Can you work these out from the model? Positions are in its coordinate system, mm. A direction names the side the tool comes from. Give positions to 0.01 mm unless a question says otherwise; leave off trailing zeros. Order: outer loops, then holes, each group sorted by start corner. A loop starts at its lowest first (then second) coordinate and runs counter-clockwise, first axis right, second up. Notation, with made-up numbers: M -28.75,-10.75 L 3.25,-10.75 A26 cw 3.25,25.25 Z; hole C -5.5,2.5 d4. An arc over 180 degrees is marked long. Use a Markdown table: item, result. Add a question column.
from build123d import *

# Parameters (mm, degrees)
SALIENTE_EXTRUIR1_DEPTH = 3
REDONDEO1_R             = 35
CROQUIS2_W              = 3
CROQUIS2_H              = 33
CORTAR_EXTRUIR1_DEPTH   = 4
CROQUIS3_W              = 11.5
CROQUIS3_H              = 13
CORTAR_EXTRUIR2_DEPTH   = 4
CROQUIS4_W              = 12
CROQUIS4_H              = 11
CORTAR_EXTRUIR3_DEPTH   = 4
REDONDEO2_R             = 10
CORTAR_EXTRUIR4_DEPTH   = 4
CROQUIS6_W              = 5
CROQUIS6_H              = 3
CORTAR_EXTRUIR5_DEPTH   = 4


with BuildPart() as part:
    # Croquis1 → Saliente-Extruir1 (new body)
    with BuildSketch(Plane.XY):
        Polygon((-21.5, 30), (-40, 30), (-95, -25), (-95, -30), (-21.5, -30), (-18.5, -30), (95, -30), (95, 30), (-18.5, 30), align=None)
    extrude(amount=SALIENTE_EXTRUIR1_DEPTH)

    # Redondeo1
    redondeo1_edges = [part.edges().sort_by_distance(p)[0] for p in [
        (95, 30, 1.5),
    ]]
    fillet(redondeo1_edges, radius=REDONDEO1_R)

    # Croquis2 → Cortar-Extruir1 (cut, through all)
    with BuildSketch(Plane.XY.offset(3)):
        with Locations((33.5, 13.5)):
            Rectangle(CROQUIS2_W, CROQUIS2_H)
        with Locations((-25.7, 13.5)):
            Rectangle(CROQUIS2_W, CROQUIS2_H)
    extrude(amount=-CORTAR_EXTRUIR1_DEPTH, mode=Mode.SUBTRACT)

    # Croquis3 → Cortar-Extruir2 (cut, through all)
    with BuildSketch(Plane(origin=(0, 0, 0), x_dir=(-1, 0, 0), z_dir=(0, 0, -1))):
        with Locations((-51, -13)):
            Rectangle(CROQUIS3_W, CROQUIS3_H)
    extrude(amount=-CORTAR_EXTRUIR2_DEPTH, mode=Mode.SUBTRACT)

    # Croquis4 → Cortar-Extruir3 (cut, through all)
    with BuildSketch(Plane(origin=(0, 0, 0), x_dir=(-1, 0, 0), z_dir=(0, 0, -1))):
        with Locations((-51, 17.5)):
            Rectangle(CROQUIS4_W, CROQUIS4_H)
    extrude(amount=-CORTAR_EXTRUIR3_DEPTH, mode=Mode.SUBTRACT)

    # Redondeo2
    redondeo2_edges = [part.edges().sort_by_distance(p)[0] for p in [
        (-40, 30, 1.5),
    ]]
    fillet(redondeo2_edges, radius=REDONDEO2_R)

    # Croquis5 → Cortar-Extruir4 (cut, through all)
    with BuildSketch(Plane(origin=(0, 0, 0), x_dir=(-1, 0, 0), z_dir=(0, 0, -1))):
        Polygon((47.171572875, 17.171572875), (45.050252532, 15.050252532), (49.292893219, 10.807611845), (51.414213562, 12.928932188), align=None)
        Polygon((85.100505063, -20.757359313), (82.97918472, -22.878679656), (78.736544033, -18.636038969), (80.857864376, -16.514718626), align=None)
    extrude(amount=-CORTAR_EXTRUIR4_DEPTH, mode=Mode.SUBTRACT)

    # Croquis6 → Cortar-Extruir5 (cut, through all)
    with BuildSketch(Plane(origin=(0, 0, 0), x_dir=(-1, 0, 0), z_dir=(0, 0, -1))):
        with Locations((32.7, 20.61)):
            Rectangle(CROQUIS6_W, CROQUIS6_H)
    extrude(amount=-CORTAR_EXTRUIR5_DEPTH, mode=Mode.SUBTRACT)


solid = part.part
1. If we section it at D-D, the plane x = -63.5: List the corners of the cut face in (y, z) for me.
2. If we section it at C-C, the plane z = 0.75: State how many separate pieces and enclosed holes the cut face has, then the cut area to 3 significant figures.
3. We'd pull the mould along Y, two halves only. Please class faces 4 (the face through (45, 17, 1)), 5 (the face through (35, 13, 2)), 6 (the face through (-69, 1, 1)): +Y half, -Y half, draft (parallel to the pull), parting line (faces both ways), or undercut.
4. If we section it at B-B, the plane y = 7.5: List the corners of the cut face in (x, z) for me, then the cut area to 3 significant figures.
5. Will these pins go through, and if not, where does the flat tip stop? pin 1 (1.5 mm diameter, centred on y = 11, z = 2, fed in from -X); pin 2 (0.9 mm diameter, centred on x = -26.5, z = 1, fed in from +Y); pin 3 (1 mm diameter, centred on y = 2.5, z = 1.5, fed in from +X).
6. On a 3-axis mill with a long thin cutter (end or side, diameter ignored), from which of +Z, -Z, +X, -X, +Y, -Y can I reach the whole of each face in a straight line? I mean faces 1 (the face through (-27.2, 13, 2)), 2 (the face through (51, 23, 1)), 3 (the face through (-39.735, 29.218, 1.521)). Say none if no direction works.
7. I need wall thicknesses on L1, parallel to X at y = -13, z = 0.95; L2, parallel to X at y = 22.5, z = 1.8; L3, parallel to X at y = 8.5, z = 2.25. Which ranges of each line are inside material? Lowest first, please. Write a range as [from, to].
8. If we section it at A-A, the plane x = 55: List the corners of the cut face in (y, z) for me, then the cut area to 3 significant figures.
Geometry results:
| question | item | result |
|---|---|---|
| 1 | outline | M -30,0 L 6.5,0 L 6.5,3 L -30,3 Z |
| 2 | separate pieces | 1 |
| 2 | enclosed holes | 5 |
| 2 | area | 9,090 mm^2 |
| 3 | face 4 | undercut |
| 3 | face 5 | draft |
| 3 | face 6 | +Y half |
| 4 | outline | M -62.5,0 L -27.2,0 L -27.2,3 L -62.5,3 Z; M -24.2,0 L 32,0 L 32,3 L -24.2,3 Z; M 35,0 L 92.69,0 L 92.69,3 L 35,3 Z |
| 4 | area | 448 mm^2 |
| 5 | pin 1 | stops at x = -59.75 |
| 5 | pin 2 | stops at y = -3 |
| 5 | pin 3 | stops at x = 94.29 |
| 6 | face 1 | +Z, -Z, +Y |
| 6 | face 2 | +Z, -Z |
| 6 | face 3 | +Z, -Z, -X, +Y |
| 7 | L1 | x = [-83, 45.25], [56.75, 95] |
| 7 | L2 | x = [-47.5, -27.2], [-24.2, 32], [35, 45], [57, 81.65] |
| 7 | L3 | x = [-61.5, -27.2], [-24.2, 32], [35, 92.29] |
| 8 | outline | M -30,0 L -19.5,0 L -19.5,3 L -30,3 Z; M -6.5,0 L 12,0 L 12,3 L -6.5,3 Z; M 23,0 L 30,0 L 30,3 L 23,3 Z |
| 8 | area | 108 mm^2 |
